Job drawing, mm, ordinate dimensions from the low corner. One solid piece. Coordinates: 2 decimals unless noted, no trailing zeros. Loops run counter-clockwise (first coordinate to the right, second up) from the corner with the lowest first, then second, coordinate; pieces in that order, holes last. Notation, with made-up numbers: (64.25, 48.25) - (101.25, 48.25) arc R32 cw to (101.25, 83.25) - close; hole circle Ø9 at (14.5, 39). An arc over 180 degrees is marked (long way). Use a Markdown table: item, result. Add a question column.
1) Band-saw the part on A-A (x = 25). Give the cut face in (y, z).
2) Pull direction X, two halves, no side cores. Call the marked faces 1, 2 and 3: +X half, -X half, draft (parallel to the pull), parting line (faces both ways), or undercut.
3) Band-saw the part on D-D (y = 15.5). Give the cut face in (x, z).
4) Band-saw the part on C-C (z = 6). Give the cut face in (x, y), plus the area to 3 significant figures.
5) Band-saw the part on B-B (y = 73). Give the cut face in (x, z), plus the area to 3 significant figures.
6) Drop flat-ended pins along their axis: P1, Ø5, axis at x = 28, y = 76.5, coming from the -Z side; P2, Ø4, axis at x = 40, y = 13, coming from the +Z side; P3, Ø1, axis at y = 69, z = 2, coming from the +X side. Give the stop position or say it passes through.
7) Probe probe 1 along Y at (x, z) = (25, 9.15); probe 2 along Y at (x, z) = (37.5, 9.25); probe 3 along Z at (x, y) = (31, 78). List the from-to ranges inside material, lowest first. Write a range as [from, to].
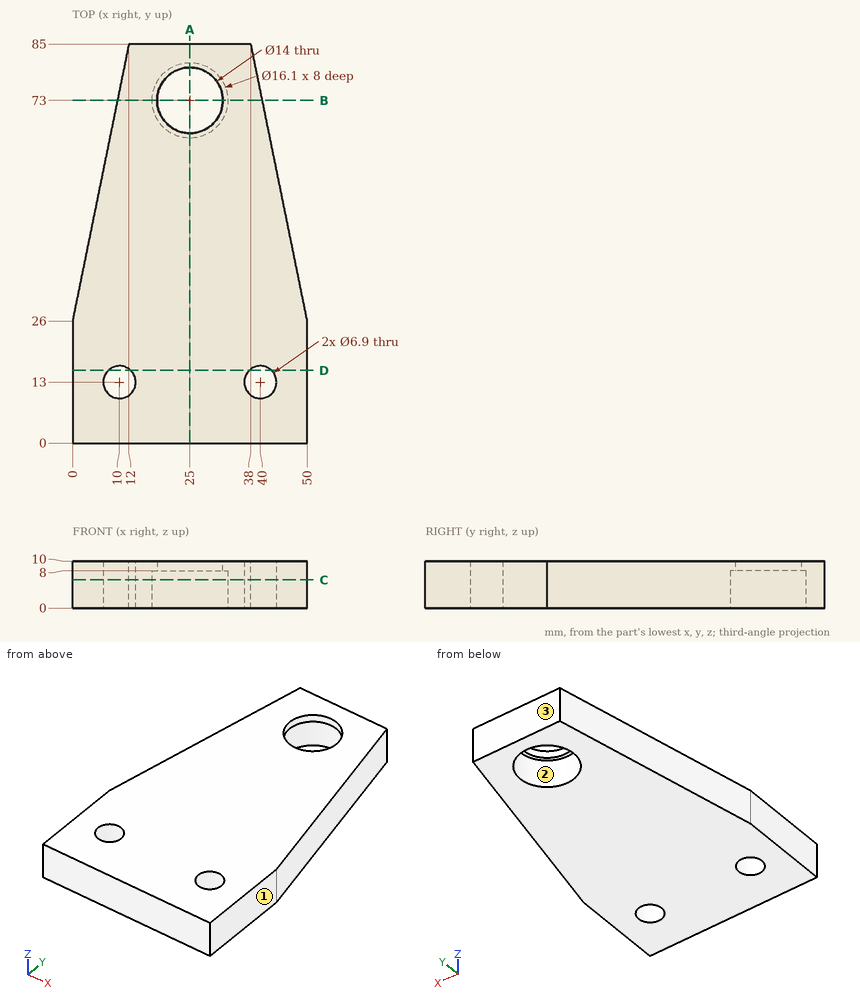
Answer block:
| question | item | result |
|---|---|---|
| 1 | outline | (0, 0) - (64.95, 0) - (64.95, 8) - (66, 8) - (66, 10) - (0, 10) - close; (80, 8) - (81.05, 8) - (81.05, 0) - (85, 0) - (85, 10) - (80, 10) - close |
| 2 | face 1 | +X half |
| 2 | face 2 | undercut |
| 2 | face 3 | draft |
| 3 | outline | (0, 0) - (7.62, 0) - (7.62, 10) - (0, 10) - close; (12.38, 0) - (37.62, 0) - (37.62, 10) - (12.38, 10) - close; (42.38, 0) - (50, 0) - (50, 10) - (42.38, 10) - close |
| 4 | outline | (0, 0) - (50, 0) - (50, 26) - (38, 85) - (12, 85) - (0, 26) - close; hole circle Ø6.9 at (10, 13); hole circle Ø16.1 at (25, 73); hole circle Ø6.9 at (40, 13) |
| 4 | area | 3,260 mm2 |
| 5 | outline | (9.56, 0) - (16.95, 0) - (16.95, 8) - (18, 8) - (18, 10) - (9.56, 10) - close; (32, 8) - (33.05, 8) - (33.05, 0) - (40.44, 0) - (40.44, 10) - (32, 10) - close |
| 5 | area | 152 mm2 |
| 6 | P1 | z = 8 |
| 6 | P2 | through |
| 6 | P3 | x = 41.36 |
| 7 | probe 1 | [0, 66], [80, 85] |
| 7 | probe 2 | [0, 10.62], [15.38, 85] |
| 7 | probe 3 | [8, 10] |
